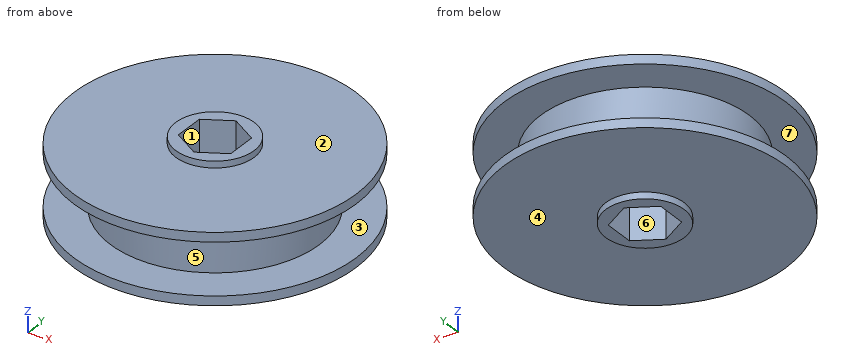
from build123d import *

# Parameters (mm, degrees)
SKETCH2_R           = 25.4
BOSS_EXTRUDE3_DEPTH = 8.21055
SKETCH3_R           = 34.29
BOSS_EXTRUDE4_DEPTH = 1.93675
SKETCH4_R           = 34.29
SKETCH4_R_2         = 9.525
CUT_EXTRUDE1_DEPTH  = 1.5875


with BuildPart() as part:
    # Sketch2 → Boss-Extrude3 (new, symmetric)
    with BuildSketch(Plane.XY):
        Circle(SKETCH2_R)
        Polygon((0, 7.332348419), (-6.35, 3.666174209), (-6.35, -3.666174209), (0, -7.332348419), (6.35, -3.666174209), (6.35, 3.666174209), align=None, mode=Mode.SUBTRACT)
    extrude(amount=BOSS_EXTRUDE3_DEPTH, both=True)

    # Sketch3 → Boss-Extrude4 (add, symmetric)
    with BuildSketch(Plane.XY.offset(8.21055)):
        Circle(SKETCH3_R)
        Polygon((0, 7.332348419), (-6.35, 3.666174209), (-6.35, -3.666174209), (0, -7.332348419), (6.35, -3.666174209), (6.35, 3.666174209), align=None, mode=Mode.SUBTRACT)
    boss_extrude4 = extrude(amount=BOSS_EXTRUDE4_DEPTH, both=True)

    # Sketch4 → Cut-Extrude1 (cut)
    with BuildSketch(Plane.XY.offset(10.1473)):
        Circle(SKETCH4_R)
        Circle(SKETCH4_R_2, mode=Mode.SUBTRACT)
    cut_extrude1 = extrude(amount=-CUT_EXTRUDE1_DEPTH, mode=Mode.SUBTRACT)

    # Mirror1: Boss-Extrude4, Cut-Extrude1 across plane
    add(boss_extrude4.mirror(Plane.XY))
    add(cut_extrude1.mirror(Plane.XY), mode=Mode.SUBTRACT)


solid = part.part
Build history of the part. All positions in model axes, mm. Face numbers are marked on the shaded views. A direction names the side the tool comes from. Coordinates: 2 decimals unless noted, no trailing zeros. Order: outer loops, then holes, each group sorted by start corner. A loop starts at its lowest first (then second) coordinate and runs counter-clockwise, first axis right, second up. Notation, with made-up numbers: M 84,86.5 L 102,86.5 A16 cw 102,98.5 Z; hole C 63,1.5 d7. An arc over 180 degrees is marked long. One line per question, with ' | ' between items. Start each with the question number.
Q1. 3-axis set-ups, long thin cutter, end or side, ignore diameter. For the marked faces 1, 2, 3 and 4: which of +Z, -Z, +X, -X, +Y, -Y reach the whole face in a straight line?
Q2. Saw through at B-B (y = 0). List the corners of the cut face in (x, z) (3 decimals).
Q3. Two-plate mould, pull along X, no slides. Class the marked faces 5, 6 and 7: +X half, -X half, draft (parallel to the pull), parting line (faces both ways), or undercut.
Q4. Flat gauge pins, fed straight in: pin 1 Ø1 at (x, y) = (-1, -22) entering from -Z; pin 2 Ø2 at (x, z) = (20, 7) entering from -Y; pin 3 Ø12 at (x, z) = (-11.5, -6.5) entering from +Y. Where does each tip first touch, or does it go through?
Q5. Saw through at C-C (x = 27.5). List the corners of the cut face in (y, z).
Q6. Probe L1, parallel to Z at x = 24, y = -23; L2, parallel to Z at x = 3.5, y = 24.5; L3, parallel to X at y = 7, z = 9.25. List the from-to ranges inside material, lowest first. Write a range as from..to.
Q7. Saw through at A-A (z = -7.25). List the corners of the cut face in (x, y), then the cut area to 3 significant figures.
Q8. Saw through at D-D (y = -19). List the corners of the cut face in (x, z), then the cut area to 3 significant figures.
Check values:
1) face 1: +Z, -Z | face 2: +Z | face 3: none | face 4: -Z
2) outline: M -34.29,-8.56 L -9.525,-8.56 L -9.525,-10.147 L -6.35,-10.147 L -6.35,10.147 L -9.525,10.147 L -9.525,8.56 L -34.29,8.56 L -34.29,6.274 L -25.4,6.274 L -25.4,-6.274 L -34.29,-6.274 Z; M 6.35,-10.147 L 9.525,-10.147 L 9.525,-8.56 L 34.29,-8.56 L 34.29,-6.274 L 25.4,-6.274 L 25.4,6.274 L 34.29,6.274 L 34.29,8.56 L 9.525,8.56 L 9.525,10.147 L 6.35,10.147 Z
3) face 5: parting line | face 6: undercut | face 7: draft
4) pin 1: stops at z = -8.56 | pin 2: stops at y = -28.54 | pin 3: stops at y = 33.85
5) outline: M -20.48,-8.56 L 20.48,-8.56 L 20.48,-6.27 L -20.48,-6.27 Z; M -20.48,6.27 L 20.48,6.27 L 20.48,8.56 L -20.48,8.56 Z
6) L1: z = -8.56..-6.27, 6.27..8.56 | L2: z = -8.56..8.56 | L3: x = -6.46..-0.58, 0.58..6.46
7) outline: C 0,0 d68.58; hole M -6.35,-3.67 L 0,-7.33 L 6.35,-3.67 L 6.35,3.67 L 0,7.33 L -6.35,3.67 Z | area: 3,550 mm2
8) outline: M -28.54,-8.56 L 28.54,-8.56 L 28.54,-6.27 L 16.86,-6.27 L 16.86,6.27 L 28.54,6.27 L 28.54,8.56 L -28.54,8.56 L -28.54,6.27 L -16.86,6.27 L -16.86,-6.27 L -28.54,-6.27 Z | area: 684 mm2
